Geometry check sheet. Reference: the model listing, model coordinates, mm. A direction names the side the tool comes from. Give positions to 0.01 mm unless a question says otherwise; leave off trailing zeros. Write each loop counter-clockwise with the first axis right and the second up, starting at its lowest first coordinate (ties: lowest second). Pieces come first, ordered by that corner, then holes. Notation, with made-up numbers: M 74,-25.5 L 95,-25.5 A21 ccw 95,-1.5 Z; hole C -22.5,30 d8. An arc over 180 degrees is marked long. Use one line per item in the form item = value. Start each with the question number.
```python
from build123d import *

# Parameters (mm, degrees)
BOSS_EXTRUDE1_DEPTH = 63.5
SKETCH3_OUTSIDE_W   = 21.198
SKETCH3_OUTSIDE_H   = 22.18
SKETCH3_OUTSIDE_R   = 3.048
CUT_EXTRUDE1_DEPTH  = 20.32
SKETCH4_OUTSIDE_W   = 21.198
SKETCH4_OUTSIDE_H   = 22.18
SKETCH4_OUTSIDE_R   = 3.048
CUT_EXTRUDE2_DEPTH  = 15.875


with BuildPart() as part:
    # Sketch2 → Boss-Extrude1 (new body)
    with BuildSketch(Plane.XY):
        Polygon((0, 3.666174209), (-3.175, 1.833087105), (-3.175, -1.833087105), (0, -3.666174209), (3.175, -1.833087105), (3.175, 1.833087105), align=None)
    extrude(amount=BOSS_EXTRUDE1_DEPTH)

    # Sketch3 outside → Cut-Extrude1 (cut)
    with BuildSketch(Plane.XY.offset(63.5)):
        Rectangle(SKETCH3_OUTSIDE_W, SKETCH3_OUTSIDE_H)
        Circle(SKETCH3_OUTSIDE_R, mode=Mode.SUBTRACT)
    extrude(amount=-CUT_EXTRUDE1_DEPTH, mode=Mode.SUBTRACT)

    # Sketch4 outside → Cut-Extrude2 (cut)
    with BuildSketch(Plane(origin=(0, 0, 0), x_dir=(-1, 0, 0), z_dir=(0, 0, -1))):
        Rectangle(SKETCH4_OUTSIDE_W, SKETCH4_OUTSIDE_H)
        Circle(SKETCH4_OUTSIDE_R, mode=Mode.SUBTRACT)
    extrude(amount=-CUT_EXTRUDE2_DEPTH, mode=Mode.SUBTRACT)


solid = part.part
```
(1) Sectioned sample at D-D, the plane z = 6.5. Record the boundary of the cut face in (x, y).
(2) Sectioned sample at A-A, the plane y = 0. Record the boundary of the cut face in (x, z) (3 decimals), plus the area to 3 significant figures.
(3) Thickness scan on probe 1 along Z at (x, y) = (-2.25, 2.25) (3 decimals); probe 2 along Y at (x, z) = (0, 4); probe 3 along Y at (x, z) = (0.5, 37). Record the ranges inside material, lowest first. Write a range as [from, to].
(4) Depth check by flat-ended pin: pin 1 (1.5 mm diameter, centred on y = -2.5, z = 26.5, fed in from -X) (3 decimals); pin 2 (4 mm diameter, centred on y = 0, z = 51.5, fed in from -X). Enter the tip coordinate at first touch or a pass-through.
(5) Tool access check on faces 1 (the cylindrical face through (0.4, 3.02, 7.83)), 2 (the cylindrical face through (-0.4, 3.02, 53.48)), 3 (the flat face through (0, 0, 0)). Record the directions out of +Z, -Z, +X, -X, +Y, -Y that give a thin tool (end or side, any length) a straight path to the whole face; none if there is none.
(6) Sectioned sample at C-C, the plane x = 2. Record the boundary of the cut face in (y, z) (3 decimals), plus the area to 3 significant figures.
(7) Sectioned sample at B-B, the plane z = 33. Record the boundary of the cut face in (x, y) (3 decimals).
Numbers:
q1.outline = C 0,0 d6.1
q2.outline = M -3.175,15.875 L -3.048,15.875 L -3.048,0 L 3.048,0 L 3.048,15.875 L 3.175,15.875 L 3.175,43.18 L 3.048,43.18 L 3.048,63.5 L -3.048,63.5 L -3.048,43.18 L -3.175,43.18 Z
q2.area = 394 mm2
q3.probe_1 = [15.875, 43.18]
q3.probe_2 = [-3.05, 3.05]
q3.probe_3 = [-3.38, 3.38]
q4.pin_1 = -3.175
q4.pin_2 = -3.05
q5.face_1 = -Z
q5.face_2 = +Z
q5.face_3 = -Z, +X, -X, +Y, -Y
q6.outline = M -2.511,15.875 L -2.3,15.875 L -2.3,0 L 2.3,0 L 2.3,15.875 L 2.511,15.875 L 2.511,43.18 L 2.3,43.18 L 2.3,63.5 L -2.3,63.5 L -2.3,43.18 L -2.511,43.18 Z
q6.area = 304 mm2
q7.outline = M -3.175,-1.833 L 0,-3.666 L 3.175,-1.833 L 3.175,1.833 L 0,3.666 L -3.175,1.833 Z
